Autodesk Inventor part; units mm, degrees
ref_plane "Work Plane2" through (11.9595, 5.75, 400) normal (1, 0, 0) x (0, -1, 0)
ref_plane "YZ Plane" through (0, 0, 0) normal (1, 0, 0) x (0, 1, 0)
ref_plane "XZ Plane" through (0, 0, 0) normal (0, 1, 0) x (-1, 0, 0)
sketch "Sketch1" plane through (0, 0, 0) normal (0, 0, 1) x (1, 0, 0)
  circle A0 centre (0, 0) radius 13.27
  circle A1 centre (0, 0) radius 10.325
  dimension "d0" = 26.54
  dimension "d1" = 20.65
extrude "Extrusion1" add sketch "Sketch1" along normal blind 400
sketch "Sketch6" plane through (0, 0, 400) normal (0, 0, 1) x (1, 0, 0)
  line L0 (0, -5.75) -> (20, -5.75)
  line L1 (20, -5.75) -> (20, 5.75)
  line L2 (20, 5.75) -> (0, 5.75)
  line L3 (0, 5.75) -> (0, -5.75)
  point P0 (0, 0)
  point P1 (0, 0)
  dimension "d13" = 20
  dimension "d14" = 11.5
extrude "Extrusion5" cut sketch "Sketch6" against normal up to next
ref_plane "Work Plane2" through (11.9595, 5.75, 400) normal (1, 0, 0) x (0, -1, 0)
sketch "Sketch7" plane through (11.9595, 5.75, 400) normal (1, 0, 0) x (0, -1, 0)
  circle A0 centre (5.75, 375) radius 2
  line L0 (16.075, 0) -> (-4.575, 0)
  line L1 (-4.575, 400) -> (16.075, 400)
  point P0 (5.75, 400)
  point P1 (11.5, 0)
  point P2 (0, 0)
  point P3 (0, 400)
  point P4 (11.5, 400)
  dimension "d17" = 4
  dimension "d21" = 25
extrude "Extrusion6" cut sketch "Sketch7" against normal through all
properties part number "inner_sheath" material "Acetal Resin, White"
Could you check a few things on this model? Use its own coordinates, in mm. Coordinates: 2 decimals unless noted, no trailing zeros. Order: outer loops, then holes, each group sorted by start corner. A loop starts at its lowest first (then second) coordinate and runs counter-clockwise, first axis right, second up. Notation, with made-up numbers: (83.25, 35) - (100.25, 35) arc R16 cw to (100.25, 43) - close; hole circle Ø11 at (-38.75, 21). An arc over 180 degrees is marked (long way). Answer in a Markdown table with one row per item. Add a question column.
(1) If we section it at A-A, the plane x = 0: Please give me the cut outline in (y, z) (3 decimals).
(2) If we mould it in two halves opening along Y, with no side actions, what happens to faces 1 (the face through (-13.26, -0.5, 197.2)), 2 (the face through (-10, 4, 0)), 3 (the face through (-10.32, -0.37, 197.2))? For each: released by +Y, released by -Y, zero draft, split by the parting line, or undercut.
(3) Will these pins go through, and if not, where does the flat tip stop? pin 1 (3 mm diameter, centred on x = -4, z = 255, fed in from -Y); pin 2 (2 mm diameter, centred on x = -7, z = 66.5, fed in from +Y); pin 3 (2.5 mm diameter, centred on x = 10.5, z = 143.5, fed in from +Y); pin 4 (8 mm diameter, centred on x = 5.5, y = -5.5, fed in from +Z).
(4) If we section it at B-B, the plane z = 64: Please give me the cut outline in (x, y) (3 decimals), then the cut area to 3 significant figures.
(5) I need wall thicknesses on L1, parallel to Y at x = 0, z = 266.5 (3 decimals); L2, parallel to Z at x = -12.2, y = 0; L3, parallel to X at y = -8, z = 155.5. Which ranges of each line are inside material? Lowest first, please.
Results are:
| question | item | result |
|---|---|---|
| 1 | outline | (-13.27, 0) - (-10.325, 0) - (-10.325, 400) - (-13.27, 400) - close; (10.325, 0) - (13.27, 0) - (13.27, 400) - (10.325, 400) - close |
| 2 | face 1 | split by the parting line |
| 2 | face 2 | zero draft |
| 2 | face 3 | undercut |
| 3 | pin 1 | stops at y = -13.03 |
| 3 | pin 2 | stops at y = 11.84 |
| 3 | pin 3 | stops at y = 9.51 |
| 3 | pin 4 | stops at z = 400 |
| 4 | outline | (8.576, -5.75) arc R10.325 cw (long way) to (8.576, 5.75) - (11.96, 5.75) arc R13.27 ccw (long way) to (11.96, -5.75) - close |
| 4 | area | 183 mm2 |
| 5 | L1 | y = -13.27 to -10.325, 10.325 to 13.27 |
| 5 | L2 | z = 0 to 23, 27 to 400 |
| 5 | L3 | x = -10.59 to -6.53, 6.53 to 10.59 |
